from build123d import *

# Parameters (mm, degrees)
SKETCH1_R           = 100
SKETCH1_R_2         = 1.75
BOSS_EXTRUDE1_DEPTH = 1.2
SKETCH2_R           = 6
BOSS_EXTRUDE2_DEPTH = 1.2


with BuildPart() as part:
    # Sketch1 → Boss-Extrude1 (new body)
    with BuildSketch(Plane.XY):
        Circle(SKETCH1_R)
        Circle(SKETCH1_R_2, mode=Mode.SUBTRACT)
    extrude(amount=BOSS_EXTRUDE1_DEPTH)

    # Sketch2 → Boss-Extrude2 (add)
    with BuildSketch(Plane.XY.offset(1.2)):
        with Locations((-3.396039654, 75)):
            Circle(SKETCH2_R)
        with Locations((19.946448935, 72.378672689)):
            Circle(SKETCH2_R)
        with Locations((41.336440128, 62.672416603)):
            Circle(SKETCH2_R)
        with Locations((58.680132553, 46.831347716)):
            Circle(SKETCH2_R)
        with Locations((70.279804755, 26.406100221)):
            Circle(SKETCH2_R)
        with Locations((75, 3.396039654)):
            Circle(SKETCH2_R)
        with Locations((72.378672689, -19.946448935)):
            Circle(SKETCH2_R)
        with Locations((62.672416603, -41.336440128)):
            Circle(SKETCH2_R)
        with Locations((46.831347716, -58.680132553)):
            Circle(SKETCH2_R)
        with Locations((26.406100221, -70.279804755)):
            Circle(SKETCH2_R)
        with Locations((3.396039654, -75)):
            Circle(SKETCH2_R)
        with Locations((-19.946448935, -72.378672689)):
            Circle(SKETCH2_R)
        with Locations((-41.336440128, -62.672416603)):
            Circle(SKETCH2_R)
        with Locations((-58.680132553, -46.831347716)):
            Circle(SKETCH2_R)
        with Locations((-70.279804755, -26.406100221)):
            Circle(SKETCH2_R)
        with Locations((-75, -3.396039654)):
            Circle(SKETCH2_R)
        with Locations((-72.378672689, 19.946448935)):
            Circle(SKETCH2_R)
        with Locations((-62.672416603, 41.336440128)):
            Circle(SKETCH2_R)
        with Locations((-46.831347716, 58.680132553)):
            Circle(SKETCH2_R)
        with Locations((-26.406100221, 70.279804755)):
            Circle(SKETCH2_R)
        with Locations((-2.264026436, 50)):
            Circle(SKETCH2_R)
        with Locations((13.297632623, 48.252448459)):
            Circle(SKETCH2_R)
        with Locations((27.557626752, 41.781611069)):
            Circle(SKETCH2_R)
        with Locations((39.120088369, 31.220898477)):
            Circle(SKETCH2_R)
        with Locations((46.85320317, 17.604066814)):
            Circle(SKETCH2_R)
        with Locations((50, 2.264026436)):
            Circle(SKETCH2_R)
        with Locations((48.252448459, -13.297632623)):
            Circle(SKETCH2_R)
        with Locations((41.781611069, -27.557626752)):
            Circle(SKETCH2_R)
        with Locations((31.220898477, -39.120088369)):
            Circle(SKETCH2_R)
        with Locations((17.604066814, -46.85320317)):
            Circle(SKETCH2_R)
        with Locations((2.264026436, -50)):
            Circle(SKETCH2_R)
        with Locations((-13.297632623, -48.252448459)):
            Circle(SKETCH2_R)
        with Locations((-27.557626752, -41.781611069)):
            Circle(SKETCH2_R)
        with Locations((-39.120088369, -31.220898477)):
            Circle(SKETCH2_R)
        with Locations((-46.85320317, -17.604066814)):
            Circle(SKETCH2_R)
        with Locations((-50, -2.264026436)):
            Circle(SKETCH2_R)
        with Locations((-48.252448459, 13.297632623)):
            Circle(SKETCH2_R)
        with Locations((-41.781611069, 27.557626752)):
            Circle(SKETCH2_R)
        with Locations((-31.220898477, 39.120088369)):
            Circle(SKETCH2_R)
        with Locations((-17.604066814, 46.85320317)):
            Circle(SKETCH2_R)
    extrude(amount=BOSS_EXTRUDE2_DEPTH)


solid = part.part
Check sheet for the modelled part. Datum: model origin and axes. Units: mm. A direction names the side the tool comes from. Round coordinates to 2 decimals unless told otherwise and drop trailing zeros.
(1) Access from +Z, -Z, +X, -X, +Y, -Y to the whole of each face (thin tool, end or side, straight path). Record for faces 3 (the flat face through (59, 47, 2.4)), 4 (the cylindrical face through (-42.53, 15.1, 1.79)).
(2) Draft check along Y on faces 1 (the flat face through (-47, -18, 2.4)), 2 (the cylindrical face through (-23.637, 64.957, 1.792)). Enter one of: pulls with the +Y half, pulls with the -Y half, needs draft (parallel to the pull), parting line crosses it, or undercut.
(3) Scan lines: probe 1 along Y at (x, z) = (0, 0.45); probe 2 along X at (y, z) = (25, 1.65); probe 3 along Z at (x, y) = (-5.5, -89.5). Record each from-to range of solid material in increasing order.
(4) Go/stop test with flat-tipped pins: P1, Ø8, axis at x = -19.5, y = 66.5, coming from the +Z side; P2, Ø4, axis at x = 29, y = -16, coming from the +Z side; P3, Ø1, axis at x = -23.5, z = 1.5, coming from the +Y side. Record where each tip stops, or that it passes through.
Check sheet entries:
1. face 3: +Z, +X, -X, +Y, -Y
1. face 4: +Z
2. face 1: needs draft
2. face 2: undercut
3. probe 1: y = -100 to -1.75, 1.75 to 100
3. probe 2: x = -75.61 to -69.14, -47.21 to -36.35, 64.45 to 76.11
3. probe 3: z = 0 to 1.2
4. P1: stops at z = 2.4
4. P2: stops at z = 1.2
4. P3: stops at y = 97.3
